Design review of the part built by this model. Coordinates are the model's own, in mm. Give positions to 0.01 mm unless a question says otherwise; leave off trailing zeros. Write each loop counter-clockwise with the first axis right and the second up, starting at its lowest first coordinate (ties: lowest second). Pieces come first, ordered by that corner, then holes. Notation, with made-up numbers: M -40,-12.5 L -17,-12.5 A14 cw -17,5.5 Z; hole C -4.75,6 d7. An arc over 180 degrees is marked long. Use a Markdown table: item, result. Add a question column.
```python
from build123d import *

# Parameters (mm, degrees)
SKETCH_1_W               = 99
SKETCH_1_H               = 66
SKETCH_2_R               = 40
CUT_EXTRUDE_1_DEPTH      = 14.5
CUT_EXTRUDE_1_DRAFT      = -2.9
MIRROR_1_COPY_1_SKETCH_R = 40
MIRROR_1_COPY_1_DEPTH    = 14.5
MIRROR_1_COPY_1_DRAFT    = -2.9
FILLET_1_R               = 2
SKETCH_3_R               = 20
CUT_EXTRUDE_2_DEPTH      = 100


with BuildPart() as part:
    # Sketch 1 → Revolve 2 (revolve)
    with BuildSketch(Plane.XY, mode=Mode.PRIVATE) as revolve_2_sk:
        with Locations((0, 33)):
            Rectangle(SKETCH_1_W, SKETCH_1_H)
    revolve(revolve_2_sk.sketch.rotate(Axis((-49.5, 0, 0), (1, 0, 0)), 90), axis=Axis((-49.5, 0, 0), (1, 0, 0)))


with BuildPart() as cut_extrude_1_tool:
    # Sketch 2 → Cut-Extrude 1 (with draft: the straight prism first)
    with BuildSketch(Plane.ZY.offset(49.5)):
        Circle(SKETCH_2_R)
    extrude(amount=-CUT_EXTRUDE_1_DEPTH)
    # Cut-Extrude 1: the draft: its side faces are tilted about the plane it starts from
    cut_extrude_1_sides = [cut_extrude_1_tool.faces().sort_by_distance(p)[0] for p in [
        (-42.25, 0, -40),
    ]]
    draft(cut_extrude_1_sides, Plane.ZY.offset(49.5), CUT_EXTRUDE_1_DRAFT)


with BuildPart() as part_1:
    add(part.part)

    # Cut-Extrude 1: cut by cut_extrude_1_tool
    add(cut_extrude_1_tool.part, mode=Mode.SUBTRACT)


with BuildPart() as mirror_1_copy_1_tool:
    # Mirror 1 copy 1 sketch → Mirror 1 copy 1 (with draft: the straight prism first)
    with BuildSketch(Plane(origin=(49.5, 0, 0), x_dir=(0, 0, 1), z_dir=(1, 0, 0))):
        Circle(MIRROR_1_COPY_1_SKETCH_R)
    extrude(amount=-MIRROR_1_COPY_1_DEPTH)
    # Mirror 1 copy 1: the draft: its side faces are tilted about the plane it starts from
    mirror_1_copy_1_sides = [mirror_1_copy_1_tool.faces().sort_by_distance(p)[0] for p in [
        (42.25, 0, -40),
    ]]
    draft(mirror_1_copy_1_sides, Plane(origin=(49.5, 0, 0), x_dir=(0, 0, 1), z_dir=(1, 0, 0)), MIRROR_1_COPY_1_DRAFT)


with BuildPart() as part_2:
    add(part_1.part)

    # Mirror 1 copy 1: cut by mirror_1_copy_1_tool
    add(mirror_1_copy_1_tool.part, mode=Mode.SUBTRACT)

    # Fillet 1
    fillet_1_edges = [part_2.edges().sort_by_distance(p)[0] for p in [
        (49.5, 0, -40),
        (35, 0, -39.265461688),
        (-49.5, 0, -66),
        (49.5, 0, -66),
        (-35, 0, -39.265461688),
    ]]
    fillet(fillet_1_edges, radius=FILLET_1_R)

    # Sketch 3 → Cut-Extrude 2 (cut)
    with BuildSketch(Plane.ZY.offset(35)):
        Circle(SKETCH_3_R)
    extrude(amount=-CUT_EXTRUDE_2_DEPTH, mode=Mode.SUBTRACT)


solid = part_2.part
```
(1) Add section A-A on y = 0. Give the boundary of the cut face in (x, z).
(2) Add section C-C on x = 33. Give the boundary of the cut face in (y, z).
(3) Wall thickness on L1, parallel to Y at x = -17, z = 0; L2, parallel to Z at x = 22, y = -9; L3, parallel to Y at x = -43, z = 15: over which ranges is each line inside the solid? List them lowest first.
(4) For pin 1 (5 mm diameter, centred on x = 11, y = 44.5, fed in from -Z); pin 2 (22.5 mm diameter, centred on y = -12, z = 4.5, fed in from +X); pin 3 (3 mm diameter, centred on x = 8, y = 30.5, fed in from +Z); pin 4 (24 mm diameter, centred on y = 0, z = 0, fed in from -X), all flat-tipped, find the tip position at first contact; note any pin that passes through.
(5) The part is to be moulded in two halves that separate along Z. For faces 1 (the flat face through (-49.5, -29, -28)), 2 (the cylindrical face through (0.665, -19.825, 62.952)), 3 (the flat face through (-35, -16, 16)), 4 (the flat face through (35, 16, 16)), say which applies: released by +Z, released by -Z, zero draft, split by the parting line, or undercut.
From the geometry:
| question | item | result |
|---|---|---|
| 1 | outline | M -49.5,-64 A2 ccw -47.5,-66 L 47.5,-66 A2 ccw 49.5,-64 L 49.5,-41.9 A2 ccw 47.6,-39.9 L 36.9,-39.36 A2 cw 35,-37.36 L 35,-20 L -35,-20 L -35,-37.36 A2 cw -36.9,-39.36 L -49.5,-40 Z; M -49.5,40 L -36.9,39.36 A2 cw -35,37.36 L -35,20 L 35,20 L 35,37.36 A2 cw 36.9,39.36 L 47.6,39.9 A2 ccw 49.5,41.9 L 49.5,64 A2 ccw 47.5,66 L -47.5,66 A2 ccw -49.5,64 Z |
| 2 | outline | C 0,0 d132; hole C 0,0 d40 |
| 3 | L1 | y = -66 to -20, 20 to 66 |
| 3 | L2 | z = -65.38 to -17.86, 17.86 to 65.38 |
| 3 | L3 | y = -64.27 to -36.73, 36.73 to 64.27 |
| 4 | pin 1 | stops at z = -50.91 |
| 4 | pin 2 | stops at x = 35 |
| 4 | pin 3 | stops at z = 59.29 |
| 4 | pin 4 | passes through |
| 5 | face 1 | zero draft |
| 5 | face 2 | split by the parting line |
| 5 | face 3 | undercut |
| 5 | face 4 | undercut |
